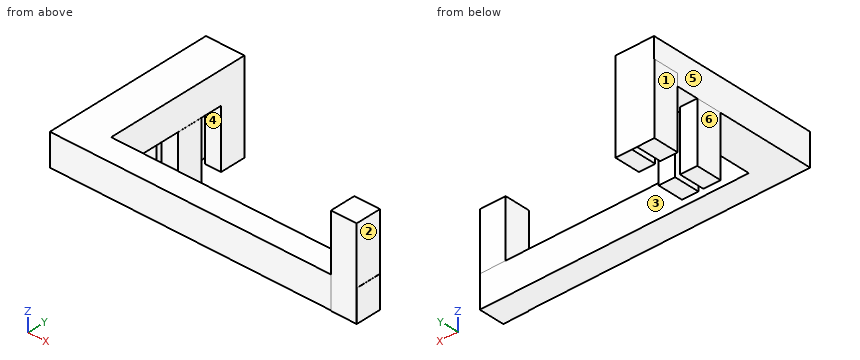
from build123d import *

# Parameters (mm, degrees)
F1_DEPTH      = 25
F2_W          = 30
F2_H          = 8.8426908478
F3_DEPTH      = 20
F5_W          = 4
F5_H          = 20
F6_DEPTH      = 46.1583091522
F6_DEPTH_BACK = 18
F7_W          = 20
F7_H          = 20
F8_DEPTH      = 70
F9_W          = 13.3632806614
F9_H          = 20
F9_W_2        = 12.7708598524
F10_DEPTH     = 47


with BuildPart() as f1:
    # F0 (on Top) → F1 (new body)
    with BuildSketch(Plane.XY):
        Polygon((120.722244599, -49.4738900023), (120.722244599, -29.9738900023), (-89.277755401, -29.9738900023), (-89.277755401, 84.3118136035), (-119.277755401, 84.3118136035), (-119.277755401, -49.6167442972), (110.722244599, -49.6167442972), (110.722244599, -49.4738900023), align=None)
    extrude(amount=F1_DEPTH)

    # F2 (on face) → F3 (join)
    with BuildSketch(Plane(origin=(0, 84.3118136035, 0), x_dir=(-1, 0, 0), z_dir=(0, 1, 0))):
        Polygon((119.5622932736, 8.8426908478), (119.277755401, 8.8426908478), (119.277755401, 0), (89.277755401, 0), (89.277755401, -46.1573091522), (119.5622932736, -46.1573091522), align=None)
        with Locations((104.277755401, 4.4213454239)):
            Rectangle(F2_W, F2_H)
    extrude(amount=-F3_DEPTH)


with BuildPart() as f1_1:
    # F4: moved
    add(f1.part.moved(Location((104, 0, 0))))

    # F5 (on Top) → F6 (cut, two sides)
    with BuildSketch(Plane.XY) as f6_sk:
        with Locations((-9.5e-08, 74.2918348312)):
            Rectangle(F5_W, F5_H)
    extrude(amount=-F6_DEPTH, mode=Mode.SUBTRACT)
    extrude(f6_sk.sketch, amount=F6_DEPTH_BACK, mode=Mode.SUBTRACT)

    # F7 (on Top) → F8 (join)
    with BuildSketch(Plane.XY):
        with Locations((214.6340256929, -40.0454027206)):
            Rectangle(F7_W, F7_H)
    extrude(amount=F8_DEPTH)

    # F9 (on Top) → F10 (join)
    with BuildSketch(Plane.XY):
        with Locations((-8.6816403307, 37.3118136035)):
            Rectangle(F9_W, F9_H)
        with Locations((8.3854299262, 37.3118136035)):
            Rectangle(F9_W_2, F9_H)
    extrude(amount=-F10_DEPTH)


solid = f1_1.part
Input: part model. Units: mm. Frame: model coordinates. Face numbers are marked on the shaded views. A direction names the side the tool comes from. Round coordinates to 2 decimals unless told otherwise and drop trailing zeros. Order: outer loops, then holes, each group sorted by start corner. A loop starts at its lowest first (then second) coordinate and runs counter-clockwise, first axis right, second up.
1. Cut plane C-C, the plane z = 13. Output: boundary loops of the cut face in (x, y).
The answers:
outline: (-15.28, -49.62) - (204.63, -49.62) - (204.63, -50.05) - (224.63, -50.05) - (224.63, -49.47) - (224.72, -49.47) - (224.72, -29.97) - (14.72, -29.97) - (14.72, 84.31) - (-15.28, 84.31) - close; hole (-2, 64.29) - (2, 64.29) - (2, 84.29) - (-2, 84.29) - close
2. Material intervals for line 1 (X direction, y = 70, z = 12.5); line 2 (Z direction, x = 38.5, y = -31); line 3 (Y direction, x = -5, z = -21), sorted ascending.
The answers:
line 1: x = -15.28 to -2, 2 to 14.72
line 2: z = 0 to 25
line 3: y = 27.31 to 47.31, 64.31 to 84.31
3. Set-up query: the marked faces 4, 5 and 6. Return all of +Z, -Z, +X, -X, +Y, -Y with unobstructed straight access to the full face (end or side cutting, diameter ignored); none if empty.
The answers:
face 4: -Z, +X, -X
face 5: +Z, -X, -Y
face 6: +Z, -Z, -X, -Y
4. Cut plane A-A, the plane z = -39. Output: boundary loops of the cut face in (x, y), then the cut area to 3 significant figures.
The answers:
outline: (-15.56, 64.31) - (-2, 64.31) - (-2, 84.29) - (2, 84.29) - (2, 64.31) - (14.72, 64.31) - (14.72, 84.31) - (-15.56, 84.31) - close; (-15.36, 27.31) - (-2, 27.31) - (-2, 47.31) - (-15.36, 47.31) - close; (2, 27.31) - (14.77, 27.31) - (14.77, 47.31) - (2, 47.31) - close
area: 1,050 mm2
5. Pin query (flat end, axial travel): P1, Ø22, axis at y = 41.5, z = -24, coming from the -X side; P2, Ø12, axis at x = 195.5, y = -34, coming from the +Z side; P3, Ø14, axis at x = 11, z = -12.5, coming from the -Y side. Return the tip coordinate at first contact, or that it passes through.
The answers:
P1: stops at x = -15.36
P2: stops at z = 25
P3: stops at y = 27.31
6. Cut plane B-B, the plane y = -33. Output: boundary loops of the cut face in (x, z), then the cut area to 3 significant figures.
The answers:
outline: (-15.28, 0) - (224.72, 0) - (224.72, 25) - (224.63, 25) - (224.63, 70) - (204.63, 70) - (204.63, 25) - (-15.28, 25) - close
area: 6,900 mm2
7. Cut plane D-D, the plane x = 46. Output: boundary loops of the cut face in (y, z), then the cut area to 3 significant figures.
The answers:
outline: (-49.62, 0) - (-29.97, 0) - (-29.97, 25) - (-49.62, 25) - close
area: 491 mm2
8. Mould query, pull axis X, two halves, no side actions, for the marked faces 1, 2 and 3. Classes: released by +X, released by -X, zero draft, split by the parting line, or undercut.
The answers:
face 1: released by -X
face 2: released by +X
face 3: zero draft
